Design review of the part built by this model. Coordinates are the model's own, in mm. A direction names the side the tool comes from. Coordinates: 2 decimals unless noted, no trailing zeros. Order: outer loops, then holes, each group sorted by start corner. A loop starts at its lowest first (then second) coordinate and runs counter-clockwise, first axis right, second up. Notation, with made-up numbers: M -12.75,33 L 36.25,33 A18 ccw 36.25,43 Z; hole C 60.25,71.25 d2. An arc over 180 degrees is marked long. Answer as a JSON object with one key per item and string values.
Autodesk Inventor part; units mm, degrees
ref_plane "YZ Plane" through (0, 0, 0) normal (1, 0, 0) x (0, 1, 0)
ref_plane "XZ Plane" through (0, 0, 0) normal (0, 1, 0) x (-1, 0, 0)
ref_plane "XY Plane" through (0, 0, 0) normal (0, 0, 1) x (1, 0, 0)
sketch "Sketch1" plane through (0, 0, 0) normal (0, 0, 1) x (1, 0, 0)
  line L0 (-110.49, 22.352) -> (110.49, 22.352)
  line L1 (110.49, 22.352) -> (110.49, -22.352)
  line L2 (110.49, -22.352) -> (-110.49, -22.352)
  line L3 (-110.49, -22.352) -> (-110.49, 22.352)
  line L4 (-110.49, 22.352) -> (110.49, -22.352) construction
  line L5 (110.49, 22.352) -> (-110.49, -22.352) construction
  line L6 (0, 22.352) -> (115.316, 22.352)
  line L7 (115.316, 22.352) -> (110.49, -22.352)
  line L8 (0, 22.352) -> (-115.316, 22.352)
  line L9 (-115.316, 22.352) -> (-110.49, -22.352)
  line L10 (119.1514, 22.352) -> (-119.1514, 22.352)
  line L11 (-119.1514, 22.352) -> (-119.1514, 24.892)
  line L12 (-119.1514, 24.892) -> (119.1514, 24.892)
  line L13 (119.1514, 24.892) -> (119.1514, 22.352)
  point P0 (0, 0)
  point P1 (0, 24.892)
  point P2 (110.49, 22.352)
  point P3 (-110.49, 22.352)
  point P4 (110.49, 22.352)
  point P5 (-115.316, 22.352)
  point P6 (115.316, 22.352)
  dimension "d0" = 220.98
  dimension "d1" = 44.704
  dimension "d2" = 115.316
  dimension "d3" = 115.316
  dimension "d10" = 2.54
  dimension "d11" = 238.3028
extrude "Extrusion1" add sketch "Sketch1" along normal blind 25.4
sketch "Sketch2" plane through (0, 0, 25.4) normal (0, 0, 1) x (1, 0, 0)
  line L0 (-120.0424, 48.8596) -> (122.5706, 48.8596)
  line L1 (122.5706, 48.8596) -> (122.5706, -0.3726)
  line L2 (122.5706, -0.3726) -> (-120.0424, -0.3726)
  line L3 (-120.0424, -0.3726) -> (-120.0424, 48.8596)
  point P0 (0, 0)
extrude "Extrusion2" [suppressed]
properties part number "Lid_Divider"
1) Add section A-A (z = 20.75). State the section outline as (x, y) points.
Taken from the geometry:
{"outline": "M -119.15,22.35 L -115.32,22.35 L -110.49,-22.35 L 110.49,-22.35 L 115.32,22.35 L 119.15,22.35 L 119.15,24.89 L -119.15,24.89 Z"}
2) Insertion check: pin 1 Ø4 at (y, z) = (-12.5, 14.5) entering from -X; pin 2 Ø3 at (y, z) = (2.5, 18.5) entering from +X; pin 3 Ø1 at (y, z) = (-8, 19) entering from -X. Each pin has a flat end and moves straight along its axis. Give the tip position at first contact, or say it passes through.
Taken from the geometry:
{"pin 1": "stops at x = -111.77", "pin 2": "stops at x = 113.33", "pin 3": "stops at x = -112.09"}
3) To check wall thickness, follow L1, parallel to X at y = 22, z = 5.5; L2, parallel to X at y = 3.5, z = 11. State the ranges of each line that lie inside material, in increasing order.
Taken from the geometry:
{"L1": "x = -115.28 to 115.28", "L2": "x = -113.28 to 113.28"}
4) Add section C-C (y = 8.5). State the section outline as (x, z) points.
Taken from the geometry:
{"outline": "M -113.82,0 L 113.82,0 L 113.82,25.4 L -113.82,25.4 Z"}
5) Add section B-B (y = -7). State the section outline as (x, z) points, and give its area (3 significant figures).
Taken from the geometry:
{"outline": "M -112.15,0 L 112.15,0 L 112.15,25.4 L -112.15,25.4 Z", "area": "5,700 mm2"}
6) Tool access review of faces 1 (the flat face through (-117, 22.352, 13)), 2 (the flat face through (-2, 24.892, 13)), 3 (the flat face through (117, 22.352, 13)): name each direction out of +Z, -Z, +X, -X, +Y, -Y from which nothing blocks a thin tool from reaching the whole face with its end or side.
Taken from the geometry:
{"face 1": "+Z, -Z, -X, -Y", "face 2": "+Z, -Z, +X, -X, +Y", "face 3": "+Z, -Z, +X, -Y"}
